```python
from build123d import *

# Parameters (mm, degrees)
SKETCH2_R           = 1
BOSS_EXTRUDE1_DEPTH = 40
CUT_EXTRUDE1_DEPTH  = 1


with BuildPart() as part:
    # Sketch1 → Revolve1 (revolve)
    with BuildSketch(Plane(origin=(0, 0, 0), x_dir=(0, 0, -1), z_dir=(1, 0, 0))):
        Polygon((0, 0), (-1.9, 0), (-1, -0.9), (-1, -1.2), (0, -1.2), align=None)
    revolve(axis=Axis((0, 0.872326939, 0), (0, -1, 0)))

    # Sketch2 → Boss-Extrude1 (add)
    with BuildSketch(Plane.XZ.offset(1.2)):
        Circle(SKETCH2_R)
    extrude(amount=BOSS_EXTRUDE1_DEPTH)

    # Sketch3 → Cut-Extrude1 (cut)
    with BuildSketch(Plane(origin=(0, 0, 0), x_dir=(1, 0, 0), z_dir=(0, 1, 0))):
        with BuildLine():
            Line((-0.9, -0.2), (-0.4, -0.2))
            ThreePointArc((-0.4, -0.2), (-0.258578644, -0.258578644), (-0.2, -0.4))
            Line((-0.2, -0.4), (-0.2, -0.9))
            Line((-0.2, -0.9), (0.2, -0.9))
            Line((0.2, -0.9), (0.2, -0.4))
            ThreePointArc((0.2, -0.4), (0.258578644, -0.258578644), (0.4, -0.2))
            Line((0.4, -0.2), (0.9, -0.2))
            Line((0.9, -0.2), (0.9, 0.2))
            Line((0.9, 0.2), (0.4, 0.2))
            ThreePointArc((0.4, 0.2), (0.258578644, 0.258578644), (0.2, 0.4))
            Line((0.2, 0.4), (0.2, 0.9))
            Line((0.2, 0.9), (-0.2, 0.9))
            Line((-0.2, 0.9), (-0.2, 0.4))
            ThreePointArc((-0.2, 0.4), (-0.258578644, 0.258578644), (-0.4, 0.2))
            Line((-0.4, 0.2), (-0.9, 0.2))
            Line((-0.9, 0.2), (-0.9, -0.2))
        make_face()
    extrude(amount=-CUT_EXTRUDE1_DEPTH, mode=Mode.SUBTRACT)


solid = part.part
```
CAD build for the part. Positions are in the model's coordinates, mm. Coordinates: 2 decimals unless noted, no trailing zeros. Order: outer loops, then holes, each group sorted by start corner. A loop starts at its lowest first (then second) coordinate and runs counter-clockwise, first axis right, second up. Notation, with made-up numbers: (3, 56.5) -> (47, 56.5) arc R30 ccw to (47, 89.5) -> close; hole circle Ø2 at (14, 15.5). An arc over 180 degrees is marked (long way). Use one line per item in the form item = value. Start each with the question number.
1) Band-saw the part on A-A on y = -26. Give the cut face in (x, z), then the cut area to 3 significant figures.
2) Drop flat-ended pins along their axis: pin 1 (0.5 mm diameter, centred on x = -0.5, z = 0, fed in from +Y); pin 2 (0.6 mm diameter, centred on y = -0.5, z = -0.5, fed in from +X); pin 3 (0.6 mm diameter, centred on x = -0.5, y = -0.5, fed in from -Z); pin 4 (1.5 mm diameter, centred on y = -29.5, z = -0.5, fed in from -X). Give the stop position or say it passes through.
3) Drill centre lines: L1, parallel to Z at x = 0.05, y = -16; L2, parallel to Y at x = 1.2, z = 0.9; L3, parallel to Z at x = -0.45, y = -17. Where is each one in solid material? Low to high. Write a range as [from, to].
4) Pull direction X, two halves, no side cores. Call faces 1 (the flat face through (0, -1, 0)), 2 (the flat face through (0.4, 0, -0.4)): +X half, -X half, draft (parallel to the pull), parting line (faces both ways), or undercut.
Entries:
q1.outline = circle Ø2 at (0, 0)
q1.area = 3.14 mm2
q2.pin_1 = 0
q2.pin_2 = 1.64
q2.pin_3 = -1.64
q2.pin_4 = -1
q3.L1 = [-1, 1]
q3.L2 = [-0.4, 0]
q3.L3 = [-0.89, 0.89]
q4.face_1 = undercut
q4.face_2 = draft
